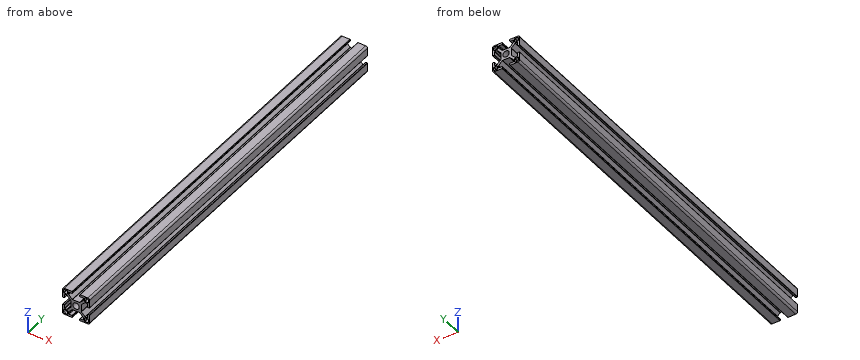
from build123d import *

# Parameters (mm, degrees)
SKETCH1_R           = 3.52998588
BOSS_EXTRUDE1_DEPTH = 228.6


with BuildPart() as part:
    # Sketch1 → Boss-Extrude1 (new, symmetric)
    with BuildSketch(Plane(origin=(0, 0, 0), x_dir=(1, 0, 0), z_dir=(0, 1, 0))):
        with BuildLine():
            Line((14.49994, -4), (13.24247465, -4))
            ThreePointArc((13.24247465, -4), (12.88892126, -4.146446609), (12.74247465, -4.5))
            Line((12.74247465, -4.5), (12.74247465, -7.732519321))
            ThreePointArc((12.74247465, -7.732519321), (12.602449697, -8.097296796), (12.242781236, -8.249967))
            Line((12.242781236, -8.249967), (10.260188032, -8.249967))
            ThreePointArc((10.260188032, -8.249967), (10.068847082, -8.211906919), (9.906636056, -8.103520976))
            Line((9.906636056, -8.103520976), (5.981117769, -4.178002689))
            ThreePointArc((5.981117769, -4.178002689), (5.872731827, -4.015791664), (5.834671745, -3.824450713))
            Line((5.834671745, -3.824450713), (5.834671745, -1.01249595))
            Line((5.834671745, -1.01249595), (5.834671745, 0.88749645))
            Line((5.834671745, 0.88749645), (5.834671745, 3.824450713))
            ThreePointArc((5.834671745, 3.824450713), (5.872731827, 4.015791664), (5.981117769, 4.178002689))
            Line((5.981117769, 4.178002689), (9.906636056, 8.103520976))
            ThreePointArc((9.906636056, 8.103520976), (10.068847082, 8.211906919), (10.260188032, 8.249967))
            Line((10.260188032, 8.249967), (12.242781236, 8.249967))
            ThreePointArc((12.242781236, 8.249967), (12.602449697, 8.097296796), (12.74247465, 7.732519321))
            Line((12.74247465, 7.732519321), (12.74247465, 4.5))
            ThreePointArc((12.74247465, 4.5), (12.88892126, 4.146446609), (13.24247465, 4))
            Line((13.24247465, 4), (14.49994, 4))
            ThreePointArc((14.49994, 4), (14.853493391, 4.146446609), (14.99994, 4.5))
            Line((14.99994, 4.5), (14.99994, 12.999948))
            ThreePointArc((14.99994, 12.999948), (14.414155906, 14.414155906), (12.999948, 14.99994))
            Line((12.999948, 14.99994), (4.5, 14.99994))
            ThreePointArc((4.5, 14.99994), (4.146446609, 14.853493391), (4, 14.49994))
            Line((4, 14.49994), (4, 13.24247465))
            ThreePointArc((4, 13.24247465), (4.146446609, 12.88892126), (4.5, 12.74247465))
            Line((4.5, 12.74247465), (7.732519321, 12.74247465))
            ThreePointArc((7.732519321, 12.74247465), (8.097296796, 12.602449697), (8.249967, 12.242781236))
            Line((8.249967, 12.242781236), (8.249967, 10.260188032))
            ThreePointArc((8.249967, 10.260188032), (8.211906919, 10.068847082), (8.103520976, 9.906636056))
            Line((8.103520976, 9.906636056), (4.178002689, 5.981117769))
            ThreePointArc((4.178002689, 5.981117769), (4.015791664, 5.872731827), (3.824450713, 5.834671745))
            Line((3.824450713, 5.834671745), (0.9499962, 5.834671745))
            Line((0.9499962, 5.834671745), (-0.9499962, 5.834671745))
            Line((-0.9499962, 5.834671745), (-3.824450713, 5.834671745))
            ThreePointArc((-3.824450713, 5.834671745), (-4.015791664, 5.872731827), (-4.178002689, 5.981117769))
            Line((-4.178002689, 5.981117769), (-8.103520976, 9.906636056))
            ThreePointArc((-8.103520976, 9.906636056), (-8.211906919, 10.068847082), (-8.249967, 10.260188032))
            Line((-8.249967, 10.260188032), (-8.249967, 12.242781236))
            ThreePointArc((-8.249967, 12.242781236), (-8.097296796, 12.602449697), (-7.732519321, 12.74247465))
            Line((-7.732519321, 12.74247465), (-4.5, 12.74247465))
            ThreePointArc((-4.5, 12.74247465), (-4.146446609, 12.88892126), (-4, 13.24247465))
            Line((-4, 13.24247465), (-4, 14.49994))
            ThreePointArc((-4, 14.49994), (-4.146446609, 14.853493391), (-4.5, 14.99994))
            Line((-4.5, 14.99994), (-12.999948, 14.99994))
            ThreePointArc((-12.999948, 14.99994), (-14.414155906, 14.414155906), (-14.99994, 12.999948))
            Line((-14.99994, 12.999948), (-14.99994, 4.5))
            ThreePointArc((-14.99994, 4.5), (-14.853493391, 4.146446609), (-14.49994, 4))
            Line((-14.49994, 4), (-13.24247465, 4))
            ThreePointArc((-13.24247465, 4), (-12.88892126, 4.146446609), (-12.74247465, 4.5))
            Line((-12.74247465, 4.5), (-12.74247465, 7.732519321))
            ThreePointArc((-12.74247465, 7.732519321), (-12.602449697, 8.097296796), (-12.242781236, 8.249967))
            Line((-12.242781236, 8.249967), (-10.260188032, 8.249967))
            ThreePointArc((-10.260188032, 8.249967), (-10.068847082, 8.211906919), (-9.906636056, 8.103520976))
            Line((-9.906636056, 8.103520976), (-5.981117769, 4.178002689))
            ThreePointArc((-5.981117769, 4.178002689), (-5.872731827, 4.015791664), (-5.834671745, 3.824450713))
            Line((-5.834671745, 3.824450713), (-5.834671745, 0.88749645))
            Line((-5.834671745, 0.88749645), (-5.834671745, -1.01249595))
            Line((-5.834671745, -1.01249595), (-5.834671745, -3.824450713))
            ThreePointArc((-5.834671745, -3.824450713), (-5.872731827, -4.015791664), (-5.981117769, -4.178002689))
            Line((-5.981117769, -4.178002689), (-9.906636056, -8.103520976))
            ThreePointArc((-9.906636056, -8.103520976), (-10.068847082, -8.211906919), (-10.260188032, -8.249967))
            Line((-10.260188032, -8.249967), (-12.242781236, -8.249967))
            ThreePointArc((-12.242781236, -8.249967), (-12.602449697, -8.097296796), (-12.74247465, -7.732519321))
            Line((-12.74247465, -7.732519321), (-12.74247465, -4.5))
            ThreePointArc((-12.74247465, -4.5), (-12.88892126, -4.146446609), (-13.24247465, -4))
            Line((-13.24247465, -4), (-14.49994, -4))
            ThreePointArc((-14.49994, -4), (-14.853493391, -4.146446609), (-14.99994, -4.5))
            Line((-14.99994, -4.5), (-14.99994, -12.999948))
            ThreePointArc((-14.99994, -12.999948), (-14.414155906, -14.414155906), (-12.999948, -14.99994))
            Line((-12.999948, -14.99994), (-4.5, -14.99994))
            ThreePointArc((-4.5, -14.99994), (-4.146446609, -14.853493391), (-4, -14.49994))
            Line((-4, -14.49994), (-4, -13.24247465))
            ThreePointArc((-4, -13.24247465), (-4.146446609, -12.88892126), (-4.5, -12.74247465))
            Line((-4.5, -12.74247465), (-7.732519321, -12.74247465))
            ThreePointArc((-7.732519321, -12.74247465), (-8.097296796, -12.602449697), (-8.249967, -12.242781236))
            Line((-8.249967, -12.242781236), (-8.249967, -10.260188032))
            ThreePointArc((-8.249967, -10.260188032), (-8.211906919, -10.068847082), (-8.103520976, -9.906636056))
            Line((-8.103520976, -9.906636056), (-4.178002689, -5.981117769))
            ThreePointArc((-4.178002689, -5.981117769), (-4.015791664, -5.872731827), (-3.824450713, -5.834671745))
            Line((-3.824450713, -5.834671745), (-0.9499962, -5.834671745))
            Line((-0.9499962, -5.834671745), (0.9499962, -5.834671745))
            Line((0.9499962, -5.834671745), (3.824450713, -5.834671745))
            ThreePointArc((3.824450713, -5.834671745), (4.015791664, -5.872731827), (4.178002689, -5.981117769))
            Line((4.178002689, -5.981117769), (8.103520976, -9.906636056))
            ThreePointArc((8.103520976, -9.906636056), (8.211906919, -10.068847082), (8.249967, -10.260188032))
            Line((8.249967, -10.260188032), (8.249967, -12.242781236))
            ThreePointArc((8.249967, -12.242781236), (8.097296796, -12.602449697), (7.732519321, -12.74247465))
            Line((7.732519321, -12.74247465), (4.5, -12.74247465))
            ThreePointArc((4.5, -12.74247465), (4.146446609, -12.88892126), (4, -13.24247465))
            Line((4, -13.24247465), (4, -14.49994))
            ThreePointArc((4, -14.49994), (4.146446609, -14.853493391), (4.5, -14.99994))
            Line((4.5, -14.99994), (12.999948, -14.99994))
            ThreePointArc((12.999948, -14.99994), (14.414155906, -14.414155906), (14.99994, -12.999948))
            Line((14.99994, -12.999948), (14.99994, -4.5))
            ThreePointArc((14.99994, -4.5), (14.853493391, -4.146446609), (14.49994, -4))
        make_face()
        with Locations(Location((0, 0, 0), (0, 0, 270))):
            Circle(SKETCH1_R, mode=Mode.SUBTRACT)
        with BuildLine():
            Line((-12.6999492, -13.6999452), (-9.880960476, -13.6999452))
            ThreePointArc((-9.880960476, -13.6999452), (-9.61155387, -13.58835333), (-9.499962, -13.318946724))
            Line((-9.499962, -13.318946724), (-9.499962, -9.87996048))
            ThreePointArc((-9.499962, -9.87996048), (-9.611260978, -9.611260978), (-9.87996048, -9.499962))
            Line((-9.87996048, -9.499962), (-13.318946724, -9.499962))
            ThreePointArc((-13.318946724, -9.499962), (-13.58835333, -9.61155387), (-13.6999452, -9.880960476))
            Line((-13.6999452, -9.880960476), (-13.6999452, -12.6999492))
            ThreePointArc((-13.6999452, -12.6999492), (-13.407053153, -13.407053153), (-12.6999492, -13.6999452))
        make_face(mode=Mode.SUBTRACT)
        with BuildLine():
            Line((13.6999452, -12.6999492), (13.6999452, -9.880960476))
            ThreePointArc((13.6999452, -9.880960476), (13.58835333, -9.61155387), (13.318946724, -9.499962))
            Line((13.318946724, -9.499962), (9.87996048, -9.499962))
            ThreePointArc((9.87996048, -9.499962), (9.611260978, -9.611260978), (9.499962, -9.87996048))
            Line((9.499962, -9.87996048), (9.499962, -13.318946724))
            ThreePointArc((9.499962, -13.318946724), (9.61155387, -13.58835333), (9.880960476, -13.6999452))
            Line((9.880960476, -13.6999452), (12.6999492, -13.6999452))
            ThreePointArc((12.6999492, -13.6999452), (13.407053153, -13.407053153), (13.6999452, -12.6999492))
        make_face(mode=Mode.SUBTRACT)
        with BuildLine():
            Line((9.87996048, 9.499962), (13.318946724, 9.499962))
            ThreePointArc((13.318946724, 9.499962), (13.58835333, 9.61155387), (13.6999452, 9.880960476))
            Line((13.6999452, 9.880960476), (13.6999452, 12.6999492))
            ThreePointArc((13.6999452, 12.6999492), (13.407053153, 13.407053153), (12.6999492, 13.6999452))
            Line((12.6999492, 13.6999452), (9.880960476, 13.6999452))
            ThreePointArc((9.880960476, 13.6999452), (9.61155387, 13.58835333), (9.499962, 13.318946724))
            Line((9.499962, 13.318946724), (9.499962, 9.87996048))
            ThreePointArc((9.499962, 9.87996048), (9.611260978, 9.611260978), (9.87996048, 9.499962))
        make_face(mode=Mode.SUBTRACT)
        with BuildLine():
            Line((-13.6999452, 12.6999492), (-13.6999452, 9.880960476))
            ThreePointArc((-13.6999452, 9.880960476), (-13.58835333, 9.61155387), (-13.318946724, 9.499962))
            Line((-13.318946724, 9.499962), (-9.87996048, 9.499962))
            ThreePointArc((-9.87996048, 9.499962), (-9.611260978, 9.611260978), (-9.499962, 9.87996048))
            Line((-9.499962, 9.87996048), (-9.499962, 13.318946724))
            ThreePointArc((-9.499962, 13.318946724), (-9.61155387, 13.58835333), (-9.880960476, 13.6999452))
            Line((-9.880960476, 13.6999452), (-12.6999492, 13.6999452))
            ThreePointArc((-12.6999492, 13.6999452), (-13.407053153, 13.407053153), (-13.6999452, 12.6999492))
        make_face(mode=Mode.SUBTRACT)
    extrude(amount=BOSS_EXTRUDE1_DEPTH, both=True)


solid = part.part
Read the model definition and answer for the solid it produces. Units are mm, in the model's axes. Round coordinates to 2 decimals unless told otherwise and drop trailing zeros. Use one line per item in the form item = value. Start each with the question number.
(1) A flat-ended cylindrical pin translates along its axis: pin 1 Ø2.5 at (x, y) = (1.5, -112.5) entering from +Z. Find the tip coordinate at first contact, or state that the pin passes through.
(2) Find the intervals of material crossed by line 1 along X through (y, z) = (-85.5, 12); line 2 along X through (y, z) = (-75, 0), in increasing order. Write a range as from..to.
(3) The part is cut by section A-A (y = -198.5). Count the separate pieces of the cut face and the enclosed holes in it, then the cut area to 3 significant figures.
Checked values:
q1.pin_1 = 5.83
q2.line_1 = -15..-13.7, -9.5..-8.25, 8.25..9.5, 13.7..15
q2.line_2 = -5.83..-3.53, 3.53..5.83
q3.separate_pieces = 1
q3.enclosed_holes = 5
q3.area = 331 mm^2
